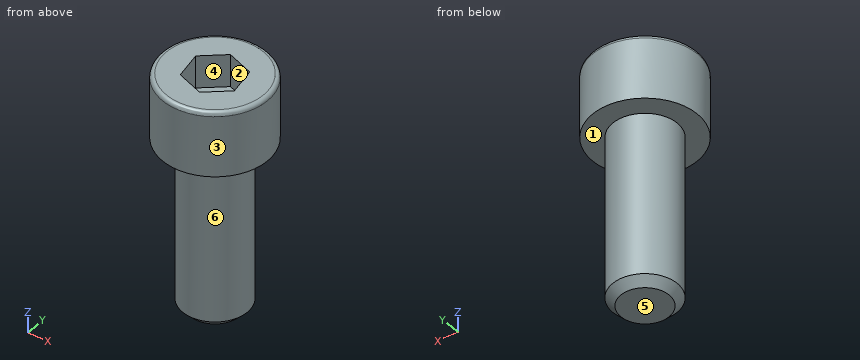
```python
from build123d import *

# Parameters (mm, degrees)
F0_R     = 6.5
F0_R_2   = 4
F1_DEPTH = 4
F2_DEPTH = 4
F3_DEPTH = 25
F4_R     = 0.5
F5_SIZE  = 1


with BuildPart() as f1:
    # F0 (on Top) → F1 (new body)
    with BuildSketch(Plane.XY):
        Circle(F0_R)
        Circle(F0_R_2, mode=Mode.SUBTRACT)
        Circle(F0_R_2)
        Polygon((-2.6272431226, -2.2577851038), (-3.2689208174, 1.1463667342), (-0.6416776948, 3.404151838), (2.6272431226, 2.2577851038), (3.2689208174, -1.1463667342), (0.6416776948, -3.404151838), align=None, mode=Mode.SUBTRACT)
        Polygon((-0.6416776948, 3.404151838), (-3.2689208174, 1.1463667342), (-2.6272431226, -2.2577851038), (0.6416776948, -3.404151838), (3.2689208174, -1.1463667342), (2.6272431226, 2.2577851038), align=None)
    extrude(amount=-F1_DEPTH)

    # F0 (on Top) → F2 (join)
    with BuildSketch(Plane.XY):
        Circle(F0_R)
        Circle(F0_R_2, mode=Mode.SUBTRACT)
        Circle(F0_R_2)
        Polygon((-2.6272431226, -2.2577851038), (-3.2689208174, 1.1463667342), (-0.6416776948, 3.404151838), (2.6272431226, 2.2577851038), (3.2689208174, -1.1463667342), (0.6416776948, -3.404151838), align=None, mode=Mode.SUBTRACT)
    extrude(amount=F2_DEPTH)

    # F0 (on Top) → F3 (join)
    with BuildSketch(Plane.XY):
        Circle(F0_R_2)
        Polygon((-2.6272431226, -2.2577851038), (-3.2689208174, 1.1463667342), (-0.6416776948, 3.404151838), (2.6272431226, 2.2577851038), (3.2689208174, -1.1463667342), (0.6416776948, -3.404151838), align=None, mode=Mode.SUBTRACT)
        Polygon((-0.6416776948, 3.404151838), (-3.2689208174, 1.1463667342), (-2.6272431226, -2.2577851038), (0.6416776948, -3.404151838), (3.2689208174, -1.1463667342), (2.6272431226, 2.2577851038), align=None)
    extrude(amount=-F3_DEPTH)

    # F4
    f4_edges = [f1.edges().sort_by_distance(p)[0] for p in [
        (-6.5, 0, 4),
    ]]
    fillet(f4_edges, radius=F4_R)

    # F5
    f5_edges = [f1.edges().sort_by_distance(p)[0] for p in [
        (-4, 0, -25),
    ]]
    chamfer(f5_edges, length=F5_SIZE)


solid = f1.part
```
Build history of the part. All positions in model axes, mm. Face numbers are marked on the shaded views. A direction names the side the tool comes from. Give positions to 0.01 mm unless a question says otherwise; leave off trailing zeros. Loops run counter-clockwise (first coordinate to the right, second up) from the corner with the lowest first, then second, coordinate; pieces in that order, holes last.
1) 3-axis set-ups, long thin cutter, end or side, ignore diameter. For the marked faces 5 and 6: which of +Z, -Z, +X, -X, +Y, -Y reach the whole face in a straight line?
Values follow:
face 5: -Z, +X, -X, +Y, -Y
face 6: -Z
2) Band-saw the part on D-D on z = -19. List the corners of the cut face in (x, y), then the cut area to 3 significant figures.
Values follow:
outline: circle Ø8 at (0, 0)
area: 50.3 mm2
3) Two-plate mould, pull along Y, no slides. Class the marked faces 1, 2, 3 and 4: released by +Y, released by -Y, zero draft, split by the parting line, or undercut.
Values follow:
face 1: zero draft
face 2: undercut
face 3: split by the parting line
face 4: undercut
4) Band-saw the part on C-C on x = 0. List the corners of the cut face in (y, z), then the cut area to 3 significant figures.
Values follow:
outline: (-6.5, -4) - (-4, -4) - (-4, -24) - (-3, -25) - (3, -25) - (4, -24) - (4, -4) - (6.5, -4) - (6.5, 3.5) arc R0.5 ccw to (6, 4) - (3.18, 4) - (3.18, 0) - (-3.18, 0) - (-3.18, 4) - (-6, 4) arc R0.5 ccw to (-6.5, 3.5) - close
area: 245 mm2
5) Band-saw the part on A-A on z = 2. List the corners of the cut face in (x, y).
Values follow:
outline: circle Ø13 at (0, 0); hole (-3.27, 1.15) - (-2.63, -2.26) - (0.64, -3.4) - (3.27, -1.15) - (2.63, 2.26) - (-0.64, 3.4) - close
6) Band-saw the part on B-B on y = 0. List the corners of the cut face in (x, z), then the cut area to 3 significant figures.
Values follow:
outline: (-6.5, -4) - (-4, -4) - (-4, -24) - (-3, -25) - (3, -25) - (4, -24) - (4, -4) - (6.5, -4) - (6.5, 3.5) arc R0.5 ccw to (6, 4) - (3.05, 4) - (3.05, 0) - (-3.05, 0) - (-3.05, 4) - (-6, 4) arc R0.5 ccw to (-6.5, 3.5) - close
area: 246 mm2
7) Probe line 1 along Z through (x, y) = (1.5, -2.5); line 2 along Z through (x, y) = (5.5, -1.25); line 3 along X through (y, z) = (0.25, 0.25). List the from-to ranges inside material, lowest first.
Values follow:
line 1: z = -25 to 0
line 2: z = -4 to 4
line 3: x = -6.5 to -3.1, 3.01 to 6.5
8) Drop flat-ended pins along their axis: P1, Ø4, axis at y = 3.5, z = -13.5, coming from the +X side; P2, Ø2, axis at x = -0.5, y = 1.5, coming from the +Z side; P3, Ø1.5, axis at y = -1, z = -21, coming from the +X side. Give the stop position or say it passes through.
Values follow:
P1: stops at x = 3.71
P2: stops at z = 0
P3: stops at x = 3.99
